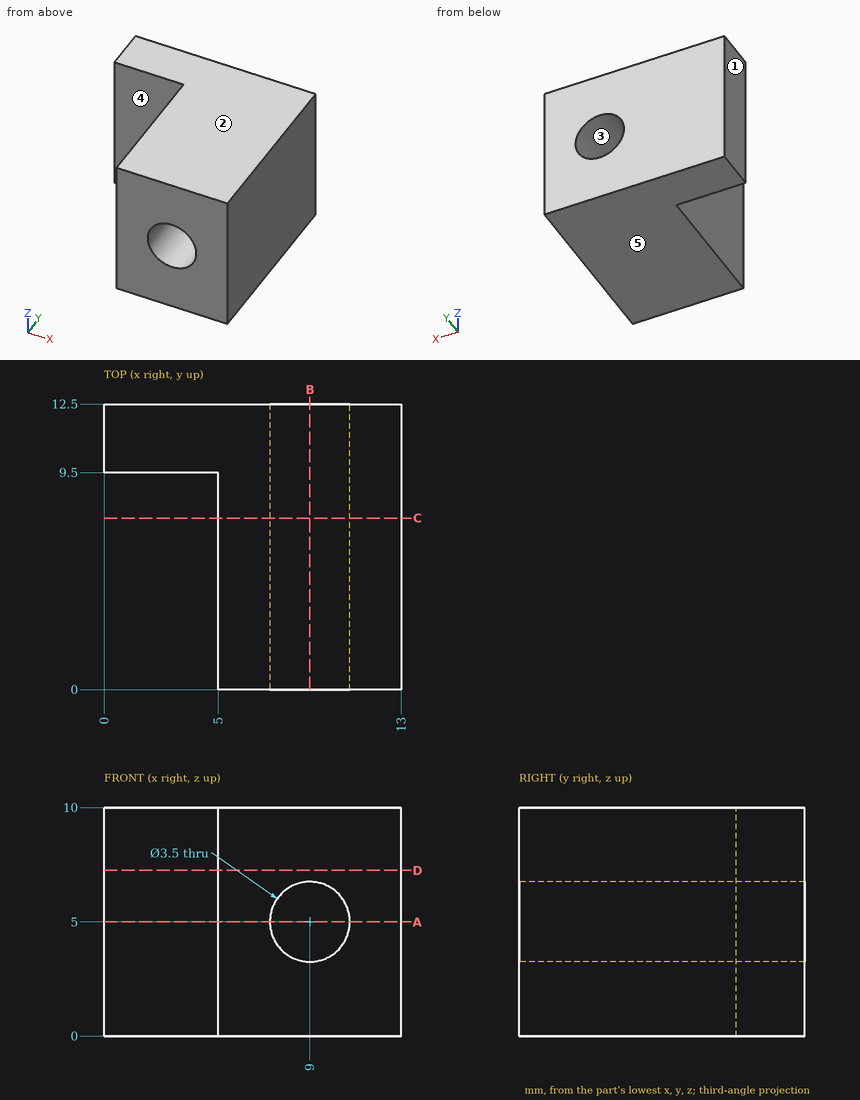
The figure shows three views and two pictorial views of one solid part (mm, origin at its lowest corner). Answer the questions. A direction names the side the tool comes from. Round coordinates to 2 decimals unless told otherwise and drop trailing zeros. Order: outer loops, then holes, each group sorted by start corner. A loop starts at its lowest first (then second) coordinate and runs counter-clockwise, first axis right, second up. Notation, with made-up numbers: (80.5, 26) -> (117.5, 26) arc R31 cw to (117.5, 56) -> close; hole circle Ø11 at (-30, 67). An arc over 180 degrees is marked (long way). Put each result on its own line as item: value.
Q1. Section B-B, the plane x = 9 is taken. Write down the section's boundary in (y, z), and give its area (4 significant figures).
Results list:
outline: (0, 0) -> (12.5, 0) -> (12.5, 3.25) -> (0, 3.25) -> close; (0, 6.75) -> (12.5, 6.75) -> (12.5, 10) -> (0, 10) -> close
area: 81.25 mm^2
Q2. Determine the mould class of the marked faces 1, 2 and 3 for opening direction Z: pulls with the +Z half, pulls with the -Z half, needs draft (parallel to the pull), parting line crosses it, or undercut.
Results list:
face 1: needs draft
face 2: pulls with the +Z half
face 3: undercut
Q3. Section C-C, the plane y = 7.5 is taken. Write down the section's boundary in (x, z), and give its area (3 significant figures).
Results list:
outline: (5, 0) -> (13, 0) -> (13, 10) -> (5, 10) -> close; hole circle Ø3.5 at (9, 5)
area: 70.4 mm^2
Q4. Each of these flat-tipped pins is pushed along its axis until it touches: P1, Ø2, axis at x = 3, y = 2, coming from the +Z side; P2, Ø1.5, axis at x = 2, z = 4, coming from the -Y side; P3, Ø5, axis at y = 2.5, z = 3, coming from the -X side. Where does it stop, or does it pass through?
Results list:
P1: through
P2: y = 9.5
P3: x = 5
Q5. Section D-D, the plane z = 7.25 is taken. Write down the section's boundary in (x, y), and give its area (3 significant figures).
Results list:
outline: (0, 9.5) -> (5, 9.5) -> (5, 0) -> (13, 0) -> (13, 12.5) -> (0, 12.5) -> close
area: 115 mm^2
Q6. Consider line 1 along Z through (x, y) = (9, 3.25); line 2 along X through (y, z) = (8.5, 1.5); line 3 along Y through (x, z) = (2.75, 7.5). Determine where each line is inside the solid, lowest interval first.
Results list:
line 1: 0 to 3.25, 6.75 to 10
line 2: 5 to 13
line 3: 9.5 to 12.5
Q7. Which of the six approach directions +Z, -Z, +X, -X, +Y, -Y give full straight-line access (tool end or side, diameter ignored) to the marked faces 4 and 5?
Results list:
face 4: +Z, -Z, -X, -Y
face 5: -Z, +X, -X, +Y, -Y
Q8. Section A-A, the plane z = 5 is taken. Write down the section's boundary in (x, y), and give its area (4 significant figures).
Results list:
outline: (0, 9.5) -> (5, 9.5) -> (5, 0) -> (7.25, 0) -> (7.25, 12.5) -> (0, 12.5) -> close; (10.75, 0) -> (13, 0) -> (13, 12.5) -> (10.75, 12.5) -> close
area: 71.25 mm^2
